```python
from build123d import *

# Parameters (mm, degrees)
SKETCH1_W           = 16.4
SKETCH1_H           = 14.65
BOSS_EXTRUDE1_DEPTH = 1
SKETCH2_R           = 0.75
SKETCH2_R_2         = 1.4
CUT_EXTRUDE1_DEPTH  = 23.013234656
SKETCH3_W           = 9.281589498
SKETCH3_H           = 6.821714685
BOSS_EXTRUDE2_DEPTH = 1


with BuildPart() as part:
    # Sketch1 → Boss-Extrude1 (new body)
    with BuildSketch(Plane(origin=(0, 0, 0), x_dir=(1, 0, 0), z_dir=(0, 1, 0))):
        with Locations((8.2, 7.325)):
            Rectangle(SKETCH1_W, SKETCH1_H)
    extrude(amount=BOSS_EXTRUDE1_DEPTH)

    # Sketch2 → Cut-Extrude1 (cut, through all)
    with BuildSketch(Plane(origin=(0, 1, 0), x_dir=(1, 0, 0), z_dir=(0, 1, 0))):
        with Locations(Location((1.429004383, 1.061195066, 0), (0, 0, 270))):
            Circle(SKETCH2_R)
        with Locations(Location((3.929004383, 1.061195066, 0), (0, 0, 270))):
            Circle(SKETCH2_R)
        with Locations(Location((6.429004383, 1.061195066, 0), (0, 0, 270))):
            Circle(SKETCH2_R)
        with Locations(Location((8.929004383, 1.061195066, 0), (0, 0, 270))):
            Circle(SKETCH2_R)
        with Locations(Location((11.429004383, 1.061195066, 0), (0, 0, 270))):
            Circle(SKETCH2_R)
        with Locations(Location((13.929004383, 1.061195066, 0), (0, 0, 270))):
            Circle(SKETCH2_R)
        with Locations(Location((2.7, 12.65, 0), (0, 0, 270))):
            Circle(SKETCH2_R_2)
        with Locations(Location((13.7, 12.65, 0), (0, 0, 270))):
            Circle(SKETCH2_R_2)
    extrude(amount=-CUT_EXTRUDE1_DEPTH, mode=Mode.SUBTRACT)

    # Sketch3 → Boss-Extrude2 (add)
    with BuildSketch(Plane(origin=(0, 1, 0), x_dir=(1, 0, 0), z_dir=(0, 1, 0))):
        with Locations((8.377516739, 6.602253277)):
            Rectangle(SKETCH3_W, SKETCH3_H)
    extrude(amount=BOSS_EXTRUDE2_DEPTH)


solid = part.part
```
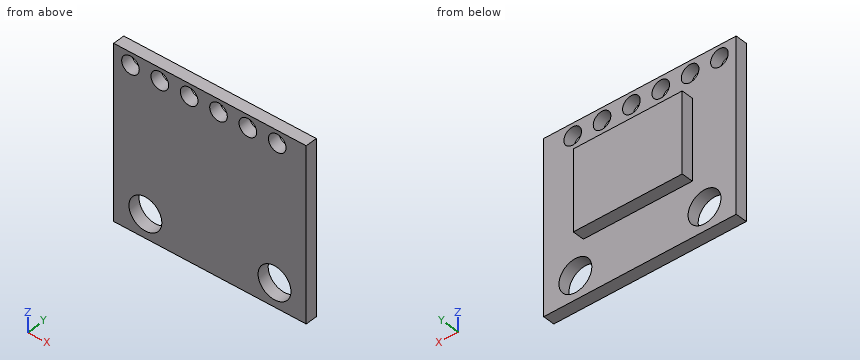
For this review, take the finished solid that the model builds, in its own axes (mm). Round coordinates to 2 decimals unless told otherwise and drop trailing zeros. Write each loop counter-clockwise with the first axis right and the second up, starting at its lowest first coordinate (ties: lowest second). Pieces come first, ordered by that corner, then holes. Notation, with made-up numbers: (10, -20) - (40, -20) arc R23 ccw to (40, -8) - close; hole circle Ø4 at (71.5, -5). An arc over 180 degrees is marked (long way). Write each question's results on one line, items separated by ' | '.
Item 1: Take a section at A-A on x = 2.7. State the section outline as (y, z) points.
Calculated:
outline: (0, -14.65) - (1, -14.65) - (1, -14.05) - (0, -14.05) - close; (0, -11.25) - (1, -11.25) - (1, 0) - (0, 0) - close
Item 2: For pin 1 (1.7 mm diameter, centred on x = 1.43, z = -1.06, fed in from +Y); pin 2 (0.5 mm diameter, centred on x = 10.5, y = 1.5, fed in from -Z); pin 3 (0.8 mm diameter, centred on x = 6.5, y = 1.5, fed in from +Z), all flat-tipped, find the tip position at first contact; note any pin that passes through.
Calculated:
pin 1: stops at y = 1 | pin 2: stops at z = -10.01 | pin 3: stops at z = -3.19
Item 3: Take a section at D-D on x = 13.7. State the section outline as (y, z) points.
Calculated:
outline: (0, -14.65) - (1, -14.65) - (1, -14.05) - (0, -14.05) - close; (0, -11.25) - (1, -11.25) - (1, -1.78) - (0, -1.78) - close; (0, -0.35) - (1, -0.35) - (1, 0) - (0, 0) - close
Item 4: To check wall thickness, follow line 1 along X through (y, z) = (0.85, -12.65); line 2 along Z through (x, y) = (2.75, 0.85); line 3 along Y through (x, z) = (7.5, -3). State the ranges of each line that lie inside material, in increasing order. Write a range as from..to.
Calculated:
line 1: x = 0..1.3, 4.1..12.3, 15.1..16.4 | line 2: z = -14.65..-14.05, -11.25..0 | line 3: y = 0..1
Item 5: Take a section at B-B on z = -6.75. State the section outline as (x, y) points, then the cut area to 3 significant figures.
Calculated:
outline: (0, 0) - (16.4, 0) - (16.4, 1) - (13.02, 1) - (13.02, 2) - (3.74, 2) - (3.74, 1) - (0, 1) - close | area: 25.7 mm^2
Item 6: Take a section at C-C on z = -12.65. State the section outline as (x, y) points.
Calculated:
outline: (0, 0) - (1.3, 0) - (1.3, 1) - (0, 1) - close; (4.1, 0) - (12.3, 0) - (12.3, 1) - (4.1, 1) - close; (15.1, 0) - (16.4, 0) - (16.4, 1) - (15.1, 1) - close
